from build123d import *

# Parameters (mm, degrees)
SKETCH2_W               = 32
SKETCH2_H               = 30
SKETCH2_W_2             = 15
BOSS_EXTRUDE1_DEPTH     = 3
SKETCH4_W               = 3
SKETCH4_H               = 30
BOSS_EXTRUDE2_DEPTH     = 3
SKETCH5_W               = 3
SKETCH5_H               = 30
BOSS_EXTRUDE3_DEPTH     = 40
CUT_EXTRUDE1_DEPTH      = 82.841309862
CUT_EXTRUDE1_DEPTH_BACK = 82.841309862
CHAMFER1_SIZE           = 10
BOSS_EXTRUDE4_DEPTH     = 375
FILLET2_R               = 10
SKETCH8_W               = 54.5
SKETCH8_H               = 30
BOSS_EXTRUDE5_DEPTH     = 4
SKETCH9_W               = 3
SKETCH9_H               = 30
BOSS_EXTRUDE6_DEPTH     = 30
CUT_EXTRUDE2_DEPTH      = 414.833625156
CUT_EXTRUDE2_DEPTH_BACK = 414.833625156
SKETCH10_R              = 1


with BuildPart() as part:
    # Sketch2 → Boss-Extrude1 (new body)
    with BuildSketch(Plane(origin=(0, 0, 0), x_dir=(1, 0, 0), z_dir=(0, 1, 0))):
        Rectangle(SKETCH2_W, SKETCH2_H)
        with Locations((-23.5, 0)):
            Rectangle(SKETCH2_W_2, SKETCH2_H)
        with Locations((23.5, 0)):
            Rectangle(SKETCH2_W_2, SKETCH2_H)
    extrude(amount=BOSS_EXTRUDE1_DEPTH)

    # Sketch4 → Boss-Extrude2 (add)
    with BuildSketch(Plane(origin=(0, 3, 0), x_dir=(1, 0, 0), z_dir=(0, 1, 0))):
        with Locations((-32.5, 0)):
            Rectangle(SKETCH4_W, SKETCH4_H)
        with Locations((32.5, 0)):
            Rectangle(SKETCH4_W, SKETCH4_H)
    extrude(amount=-BOSS_EXTRUDE2_DEPTH)

    # Sketch5 → Boss-Extrude3 (add)
    with BuildSketch(Plane(origin=(0, 3, 0), x_dir=(1, 0, 0), z_dir=(0, 1, 0))):
        with Locations((-32.5, 0)):
            Rectangle(SKETCH5_W, SKETCH5_H)
        with Locations((32.5, 0)):
            Rectangle(SKETCH5_W, SKETCH5_H)
    extrude(amount=BOSS_EXTRUDE3_DEPTH)

    # Sketch6 → Cut-Extrude1 (cut, two sides: drawn at the far end of the back side and taken through both)
    with BuildSketch(Plane.ZY.offset(34).offset(-CUT_EXTRUDE1_DEPTH_BACK)):
        with BuildLine():
            Line((-7.5, 45.5), (7.5, 45.5))
            Line((7.5, 45.5), (7.5, 40.5))
            ThreePointArc((7.5, 40.5), (0, 33), (-7.5, 40.5))
            Line((-7.5, 40.5), (-7.5, 45.5))
        make_face()
    extrude(amount=CUT_EXTRUDE1_DEPTH + CUT_EXTRUDE1_DEPTH_BACK, mode=Mode.SUBTRACT)

    # Chamfer1
    chamfer1_edges = [part.edges().sort_by_distance(p)[0] for p in [
        (-34, 0, 0),
        (34, 0, 0),
        (-31, 3, 0),
        (31, 3, 0),
    ]]
    chamfer(chamfer1_edges, length=CHAMFER1_SIZE)

    # Sketch7 → Boss-Extrude4 (add)
    with BuildSketch(Plane.XZ):
        Polygon((-24, 15), (24, 15), (24, -15.023541852), (19, -15.023541852), (19, 10), (-19, 10), (-19, -15.023541852), (-24, -15.023541852), align=None)
    extrude(amount=BOSS_EXTRUDE4_DEPTH)

    # Fillet2
    fillet2_edges = [part.edges().sort_by_distance(p)[0] for p in [
        (24, -187.5, 15),
        (-24, -187.5, 15),
    ]]
    fillet(fillet2_edges, radius=FILLET2_R)

    # Sketch8 → Boss-Extrude5 (add)
    with BuildSketch(Plane.XZ.offset(375)):
        Rectangle(SKETCH8_W, SKETCH8_H)
    extrude(amount=BOSS_EXTRUDE5_DEPTH)

    # Sketch9 → Boss-Extrude6 (add)
    with BuildSketch(Plane.XZ.offset(379)):
        with Locations((-25.75, 0)):
            Rectangle(SKETCH9_W, SKETCH9_H)
        with Locations((25.75, 0)):
            Rectangle(SKETCH9_W, SKETCH9_H)
    extrude(amount=BOSS_EXTRUDE6_DEPTH)

    # Sketch10 → Cut-Extrude2 (cut, two sides: drawn at the far end of the back side and taken through both)
    with BuildSketch(Plane.ZY.offset(27.25).offset(-CUT_EXTRUDE2_DEPTH_BACK)):
        with Locations((-12.451139345, -405.721121856)):
            Circle(SKETCH10_R)
        with Locations((11.548860655, -405.721121856)):
            Circle(SKETCH10_R)
        with Locations((-12.451139345, -381.721121856)):
            Circle(SKETCH10_R)
        with Locations((11.548860655, -381.721121856)):
            Circle(SKETCH10_R)
        with Locations((-0.451139345, -381.721121856)):
            Circle(SKETCH10_R)
    extrude(amount=CUT_EXTRUDE2_DEPTH + CUT_EXTRUDE2_DEPTH_BACK, mode=Mode.SUBTRACT)


solid = part.part
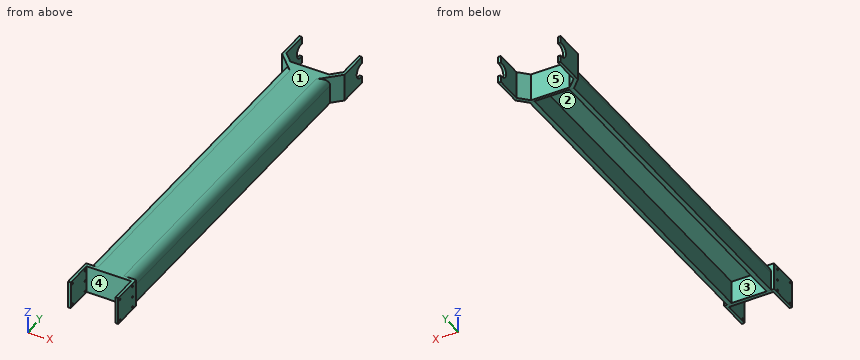
For this review, take the finished solid that the model builds, in its own axes (mm). Face numbers are marked on the shaded views. A direction names the side the tool comes from. Round coordinates to 2 decimals unless told otherwise and drop trailing zeros. Order: outer loops, then holes, each group sorted by start corner. A loop starts at its lowest first (then second) coordinate and runs counter-clockwise, first axis right, second up. Notation, with made-up numbers: M 83,36.25 L 142,36.25 A8 ccw 142,40.25 Z; hole C 6,17 d3. An arc over 180 degrees is marked long. Use a Markdown table: item, result. Add a question column.
Item 1: Tool access review of the marked faces 1 and 2: name each direction out of +Z, -Z, +X, -X, +Y, -Y from which nothing blocks a thin tool from reaching the whole face with its end or side.
Item 2: Add section A-A, the plane x = 8. Give the boundary of the cut face in (y, z), then the cut area to 4 significant figures.
Item 3: Add section B-B, the plane y = -259. Give the boundary of the cut face in (x, z).
Item 4: Mouldability with a two-part tool opening along Y and no side actions: class the marked faces 3, 4 and 5 as released by +Y, released by -Y, zero draft, split by the parting line, or undercut.
Item 5: Insertion check: pin 1 (10 mm diameter, centred on y = -26, z = 5.5, fed in from +X); pin 2 (2.5 mm diameter, centred on y = -405.72, z = 11.55, fed in from -X); pin 3 (4 mm diameter, centred on x = 22.5, z = 0.5, fed in from +Y); pin 4 (17 mm diameter, centred on x = -1, y = -393.5, fed in from -Z) (3 decimals). Each pin has a flat end and moves straight along its axis. Give the tip position at first contact, or say it passes through.
Item 6: To check wall thickness, follow line 1 along Y through (x, z) = (-2.5, -12.5); line 2 along X through (y, z) = (-296.5, -4); line 3 along X through (y, z) = (-385.5, -1.5). State the ranges of each line that lie inside material, in increasing order.
Geometry results:
| question | item | result |
|---|---|---|
| 1 | face 1 | +Z, +X, -X, +Y, -Y |
| 1 | face 2 | -Z |
| 2 | outline | M -379,-15 L -375,-15 L -375,10 L 0,10 L 0,-15 L 3,-15 L 3,15 L -379,15 Z |
| 2 | area | 2,085 mm² |
| 3 | outline | M -24,-15.02 L -19,-15.02 L -19,10 L 19,10 L 19,-15.02 L 24,-15.02 L 24,5 A10 ccw 14,15 L -14,15 A10 ccw -24,5 Z |
| 4 | face 3 | undercut |
| 4 | face 4 | released by -Y |
| 4 | face 5 | released by +Y |
| 5 | pin 1 | stops at x = 24 |
| 5 | pin 2 | stops at x = -27.25 |
| 5 | pin 3 | stops at y = 6.5 |
| 5 | pin 4 | passes through |
| 6 | line 1 | y = -379 to -375, 0 to 3 |
| 6 | line 2 | x = -24 to -19, 19 to 24 |
| 6 | line 3 | x = -27.25 to -24.25, 24.25 to 27.25 |
